Design review of the part built by this model. Coordinates are the model's own, in mm. A direction names the side the tool comes from. Round coordinates to 2 decimals unless told otherwise and drop trailing zeros. Order: outer loops, then holes, each group sorted by start corner. A loop starts at its lowest first (then second) coordinate and runs counter-clockwise, first axis right, second up. Notation, with made-up numbers: M 20.25,-8 L 66.25,-8 A19 cw 66.25,25 Z; hole C 8,83.5 d3. An arc over 180 degrees is marked long. Use a Markdown table: item, result. Add a question column.
(1) To check wall thickness, follow probe 1 along X at (y, z) = (2.3, -40); probe 2 along X at (y, z) = (1.9, -35); probe 3 along X at (y, z) = (1.7, -39). State the ranges of each line that lie inside material, in increasing order. Write a range as from..to.
(2) Take a section at A-A (x = 6). Write out the cut boundary in (y, z), then the cut area to 3 significant figures.
(3) Take a section at C-C (x = -10). Write out the cut boundary in (y, z), then the cut area to 3 significant figures.
(4) Take a section at D-D (z = -54). Write out the cut boundary in (x, y).
(5) For pin 1 (1.5 mm diameter, centred on y = 2, z = -28.5, fed in from +X), flat-tipped, find the tip position at first contact; note if it passes through.
(6) Machinability: for faces 1 (the face through (0, 2, 60.5)), 2 (the face through (24, 1, 0)), 3 (the face through (22, 2, -43.5)), which of the approach directions +Z, -Z, +X, -X, +Y, -Y give a long, thin tool a straight path to every point of the face, cutting with its end or side? Answer none if there is none.
(7) Take a section at B-B (z = 40). Write out the cut boundary in (x, y).
(8) The part is to be moulded in two halves that separate along X. For faces 4 (the face through (21, 2, -28)), 5 (the face through (17, 2, 55)), 6 (the face through (-24, 1, 1)), 7 (the face through (5, 0, -1)), say which applies: released by +X, released by -X, zero draft, split by the parting line, or undercut.
```python
from build123d import *

# Parameters (mm, degrees)
SKETCH1_W            = 48
SKETCH1_H            = 213
SKETCH1_R            = 3.2
BOSS_EXTRUDE1_DEPTH  = 3
SKETCH2_W            = 3
SKETCH2_H            = 21
SKETCH2_H_2          = 30
CUT_EXTRUDE1_DEPTH   = 110.211949896
SKETCH3_W            = 10
SKETCH3_H            = 3
CUT_EXTRUDE2_DEPTH   = 110.211949896
SKETCH4_R            = 1.3
CUT_EXTRUDE3_DEPTH   = 110.211949896
SKETCH5_W            = 48
SKETCH5_H            = 42
CUT_EXTRUDE4_DEPTH   = 110.211949896
SKETCH6_W            = 34
SKETCH6_H            = 11
CUT_EXTRUDE5_DEPTH   = 69.885775019
FILLET1_R            = 2
FILLET1_OF_MIRROR1_R = 2
SKETCH7_R            = 1.5
CUT_EXTRUDE6_DEPTH   = 69.885775019


with BuildPart() as part:
    # Sketch1 → Boss-Extrude1 (new body)
    with BuildSketch(Plane(origin=(0, 0, 0), x_dir=(1, 0, 0), z_dir=(0, 1, 0))):
        Rectangle(SKETCH1_W, SKETCH1_H)
        with Locations(Location((0, 0, 0), (0, 0, 270))):
            Circle(SKETCH1_R, mode=Mode.SUBTRACT)
    extrude(amount=BOSS_EXTRUDE1_DEPTH)

    # Sketch2 → Cut-Extrude1 (cut, through all)
    with BuildSketch(Plane(origin=(0, 3, 0), x_dir=(1, 0, 0), z_dir=(0, 1, 0))):
        with Locations((22.5, 75)):
            Rectangle(SKETCH2_W, SKETCH2_H)
        with Locations((22.5, 28.5)):
            Rectangle(SKETCH2_W, SKETCH2_H_2)
        with Locations((22.5, -28.5)):
            Rectangle(SKETCH2_W, SKETCH2_H_2)
        with Locations((22.5, -75)):
            Rectangle(SKETCH2_W, SKETCH2_H)
    extrude(amount=-CUT_EXTRUDE1_DEPTH, mode=Mode.SUBTRACT)

    # Sketch3 → Cut-Extrude2 (cut, through all)
    with BuildSketch(Plane(origin=(0, 3, 0), x_dir=(1, 0, 0), z_dir=(0, 1, 0))):
        with Locations((2.5, -21.5)):
            Rectangle(SKETCH3_W, SKETCH3_H)
        with Locations((2.5, 21.5)):
            Rectangle(SKETCH3_W, SKETCH3_H)
    extrude(amount=-CUT_EXTRUDE2_DEPTH, mode=Mode.SUBTRACT)

    # Sketch4 → Cut-Extrude3 (cut, through all)
    with BuildSketch(Plane(origin=(0, 3, 0), x_dir=(1, 0, 0), z_dir=(0, 1, 0))):
        with Locations(Location((-6.1, -35, 0), (0, 0, 270))):
            Circle(SKETCH4_R)
        with Locations(Location((-6.1, 35, 0), (0, 0, 90))):
            Circle(SKETCH4_R)
    extrude(amount=-CUT_EXTRUDE3_DEPTH, mode=Mode.SUBTRACT)

    # Sketch5 → Cut-Extrude4 (cut, through all)
    with BuildSketch(Plane(origin=(0, 3, 0), x_dir=(1, 0, 0), z_dir=(0, 1, 0))):
        with Locations((0, 85.5)):
            Rectangle(SKETCH5_W, SKETCH5_H)
        with Locations((0, -85.5)):
            Rectangle(SKETCH5_W, SKETCH5_H)
    extrude(amount=-CUT_EXTRUDE4_DEPTH, mode=Mode.SUBTRACT)

    # Sketch6 → Cut-Extrude5 (cut, through all)
    with BuildSketch(Plane(origin=(0, 3, 0), x_dir=(1, 0, 0), z_dir=(0, 1, 0))):
        with Locations((0, 55)):
            Rectangle(SKETCH6_W, SKETCH6_H)
    cut_extrude5 = extrude(amount=-CUT_EXTRUDE5_DEPTH, mode=Mode.SUBTRACT)

    # Fillet1
    fillet1_edges = [part.edges().sort_by_distance(p)[0] for p in [
        (-17, 1.5, -49.5),
        (-17, 1.5, -60.5),
        (17, 1.5, -60.5),
        (17, 1.5, -49.5),
    ]]
    fillet(fillet1_edges, radius=FILLET1_R)

    # Mirror1: Cut-Extrude5 across plane
    add(cut_extrude5.mirror(Plane.XY), mode=Mode.SUBTRACT)

    # Fillet1 of Mirror1
    fillet1_of_mirror1_edges = [part.edges().sort_by_distance(p)[0] for p in [
        (-17, 1.5, 49.5),
        (-17, 1.5, 60.5),
        (17, 1.5, 60.5),
        (17, 1.5, 49.5),
    ]]
    fillet(fillet1_of_mirror1_edges, radius=FILLET1_OF_MIRROR1_R)

    # Sketch7 → Cut-Extrude6 (cut, through all)
    with BuildSketch(Plane(origin=(0, 3, 0), x_dir=(1, 0, 0), z_dir=(0, 1, 0))):
        with Locations(Location((-14, -40, 0), (0, 0, 270))):
            Circle(SKETCH7_R)
        with Locations(Location((-4, -40, 0), (0, 0, 270))):
            Circle(SKETCH7_R)
    cut_extrude6 = extrude(amount=-CUT_EXTRUDE6_DEPTH, mode=Mode.SUBTRACT)

    # Mirror2: Cut-Extrude6 across plane
    add(cut_extrude6.mirror(Plane.XY), mode=Mode.SUBTRACT)


solid = part.part
```
Verdict:
| question | item | result |
|---|---|---|
| 1 | probe 1 | x = -24..-15.5, -12.5..-5.5, -2.5..21 |
| 1 | probe 2 | x = -24..-7.4, -4.8..21 |
| 1 | probe 3 | x = -24..-15.12, -12.88..-5.12, -2.88..21 |
| 2 | outline | M 0,-64.5 L 3,-64.5 L 3,-60.5 L 0,-60.5 Z; M 0,-49.5 L 3,-49.5 L 3,-23 L 0,-23 Z; M 0,-20 L 3,-20 L 3,20 L 0,20 Z; M 0,23 L 3,23 L 3,49.5 L 0,49.5 Z; M 0,60.5 L 3,60.5 L 3,64.5 L 0,64.5 Z |
| 2 | area | 303 mm^2 |
| 3 | outline | M 0,-64.5 L 3,-64.5 L 3,-60.5 L 0,-60.5 Z; M 0,-49.5 L 3,-49.5 L 3,49.5 L 0,49.5 Z; M 0,60.5 L 3,60.5 L 3,64.5 L 0,64.5 Z |
| 3 | area | 321 mm^2 |
| 4 | outline | M -24,0 L -17,0 L -17,3 L -24,3 Z; M 17,0 L 24,0 L 24,3 L 17,3 Z |
| 5 | pin 1 | stops at x = 21 |
| 6 | face 1 | +Y, -Y |
| 6 | face 2 | +Z, -Z, +X, +Y, -Y |
| 6 | face 3 | +X, +Y, -Y |
| 7 | outline | M -24,0 L -15.5,0 L -15.5,3 L -24,3 Z; M -12.5,0 L -5.5,0 L -5.5,3 L -12.5,3 Z; M -2.5,0 L 21,0 L 21,3 L -2.5,3 Z |
| 8 | face 4 | released by +X |
| 8 | face 5 | undercut |
| 8 | face 6 | released by -X |
| 8 | face 7 | zero draft |
